Model file for the job. Use its own axes, mm. Give positions to 0.01 mm unless a question says otherwise; leave off trailing zeros. Loops run counter-clockwise (first coordinate to the right, second up) from the corner with the lowest first, then second, coordinate; pieces in that order, holes last. Notation, with made-up numbers: M 66,68 L 85,68 A26 ccw 85,103 Z; hole C -11,46 d2. An arc over 180 degrees is marked long. Answer in a Markdown table with one row per item.
```python
from build123d import *

# Parameters (mm, degrees)
F0_R     = 127
F1_DEPTH = 127
F2_R     = 127
F3_DEPTH = 127
F4_R     = 127
F5_DEPTH = 127


with BuildPart() as f1:
    # F0 (on Front) → F1 (new body, symmetric)
    with BuildSketch(Plane.XZ):
        Circle(F0_R)
    extrude(amount=F1_DEPTH, both=True)

    # F2 (on Right) → F3 (intersect, symmetric)
    with BuildSketch(Plane.YZ):
        Circle(F2_R)
    extrude(amount=F3_DEPTH, both=True, mode=Mode.INTERSECT)

    # F4 (on Top) → F5 (intersect, symmetric)
    with BuildSketch(Plane.XY):
        Circle(F4_R)
    extrude(amount=F5_DEPTH, both=True, mode=Mode.INTERSECT)


solid = f1.part
```
Q1. Saw through at A-A (x = 64.5). Give the cut face in (y, z).
Reported:
| item | result |
|---|---|
| outline | M -109.4,-64.5 A127 ccw -64.5,-109.4 L 64.5,-109.4 A127 ccw 109.4,-64.5 L 109.4,64.5 A127 ccw 64.5,109.4 L -64.5,109.4 A127 ccw -109.4,64.5 Z |
Q2. Saw through at B-B (y = 71.5). Give the cut face in (x, z).
Reported:
| item | result |
|---|---|
| outline | M -104.96,-71.5 A127 ccw -71.5,-104.96 L 71.5,-104.96 A127 ccw 104.96,-71.5 L 104.96,71.5 A127 ccw 71.5,104.96 L -71.5,104.96 A127 ccw -104.96,71.5 Z |
Q3. Saw through at C-C (y = 111). Give the cut face in (x, z), and give its area (3 significant figures).
Reported:
| item | result |
|---|---|
| outline | M -61.71,-61.71 L 61.71,-61.71 L 61.71,61.71 L -61.71,61.71 Z |
| area | 15,200 mm² |
Q4. Probe probe 1 along Z at (x, y) = (-101, 18); probe 2 along X at (y, z) = (37.5, 82.5); probe 3 along X at (y, z) = (54.5, -55). List the from-to ranges inside material, lowest first.
Reported:
| item | result |
|---|---|
| probe 1 | -76.99 to 76.99 |
| probe 2 | -96.55 to 96.55 |
| probe 3 | -114.47 to 114.47 |
Q5. Drop flat-ended pins along their axis: pin 1 (6 mm diameter, centred on y = -76, z = -74.5, fed in from +X); pin 2 (5 mm diameter, centred on x = -82.5, y = -73.5, fed in from +Z); pin 3 (1.5 mm diameter, centred on x = -35.5, y = 61, fed in from +Z). Give the stop position or say it passes through.
Reported:
| item | result |
|---|---|
| pin 1 | x = 103.74 |
| pin 2 | z = 98.64 |
| pin 3 | z = 111.8 |
Q6. Saw through at D-D (x = -107). Give the cut face in (y, z).
Reported:
| item | result |
|---|---|
| outline | M -68.41,-68.41 L 68.41,-68.41 L 68.41,68.41 L -68.41,68.41 Z |
